Here's the drawing with two shaded views (mm, measured from the low corner). I have some questions. Coordinates: 2 decimals unless noted, no trailing zeros. Loops run counter-clockwise (first coordinate to the right, second up) from the corner with the lowest first, then second, coordinate; pieces in that order, holes last. Notation, with made-up numbers: (53.25, 10) - (57.25, 10) arc R23 cw to (57.25, 36) - close; hole circle Ø1 at (33, -31.75). An arc over 180 degrees is marked (long way). One line per item, written item: value. Start each with the question number.
(1) If I drill on line 1 along Y through (x, z) = (230, 6); line 2 along X through (y, z) = (226, 1.25); line 3 along Y through (x, z) = (124, 3.5), over which ranges is the centre line in solid material (lowest first)? Write a range as from..to.
(2) If we section it at A-A on y = 20: Write out the boundary of the cut face in (x, z).
(3) If we section it at D-D on z = 3.5: Count the separate pieces of the cut face and the enclosed holes in it, then the cut area to 3 significant figures.
(4) If we section it at B-B on y = 125: Write out the boundary of the cut face in (x, z), then the cut area to 3 significant figures.
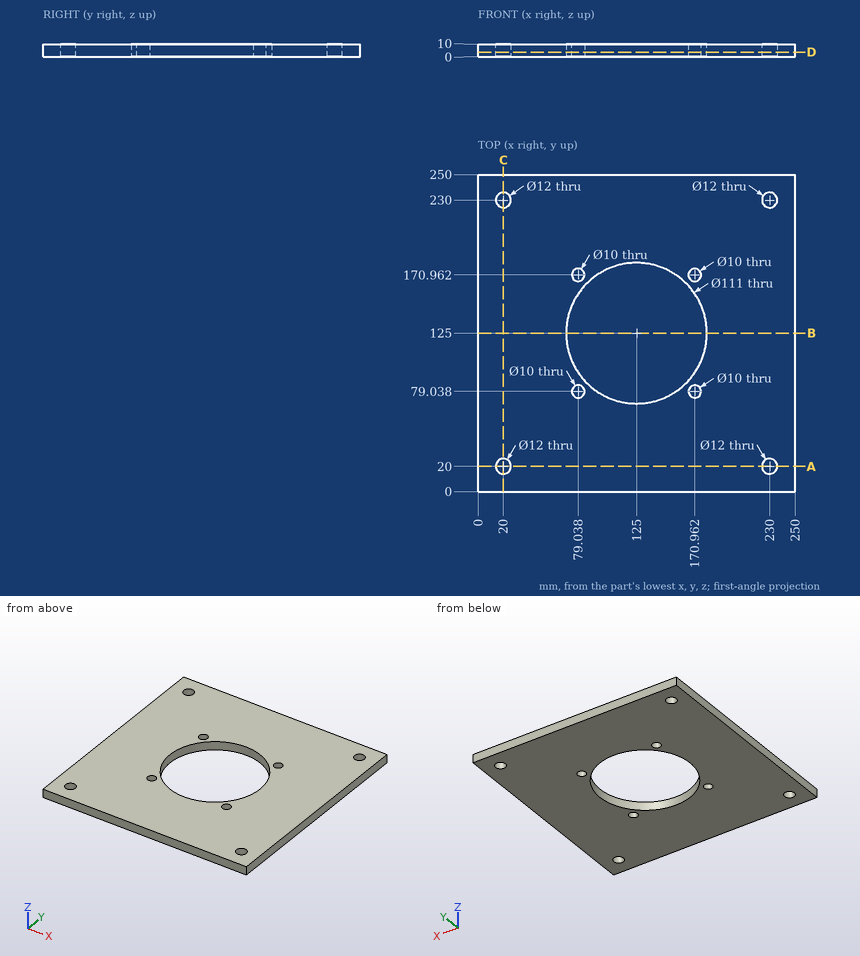
Values:
1. line 1: y = 0..14, 26..224, 236..250
1. line 2: x = 0..15.53, 24.47..225.53, 234.47..250
1. line 3: y = 0..69.51, 180.49..250
2. outline: (0, 0) - (14, 0) - (14, 10) - (0, 10) - close; (26, 0) - (224, 0) - (224, 10) - (26, 10) - close; (236, 0) - (250, 0) - (250, 10) - (236, 10) - close
3. separate pieces: 1
3. enclosed holes: 9
3. area: 52,100 mm2
4. outline: (0, 0) - (69.5, 0) - (69.5, 10) - (0, 10) - close; (180.5, 0) - (250, 0) - (250, 10) - (180.5, 10) - close
4. area: 1,390 mm2
